Check sheet for the modelled part. Datum: model origin and axes. Units: mm. Coordinates: 2 decimals unless noted, no trailing zeros. Order: outer loops, then holes, each group sorted by start corner. A loop starts at its lowest first (then second) coordinate and runs counter-clockwise, first axis right, second up.
1. Cross-section at C-C (x = 0). Enter the section's corners in (y, z) (1 decimal).
2. Cross-section at D-D (y = 190.5). Enter the section's corners in (x, z) (1 decimal), then the cut area to 3 significant figures.
3. Cross-section at A-A (z = 0). Enter the section's corners in (x, y) (1 decimal).
4. Cross-section at B-B (y = 6.35). Enter the section's corners in (x, z) (1 decimal).
5. Gauge pin test, flat ends, axial feed: pin 1 Ø1 at (y, z) = (171, -1) entering from -X; pin 2 Ø1.5 at (y, z) = (73.5, 3.5) entering from -X; pin 3 Ø1 at (x, z) = (0.5, 0.5) entering from -Y. Record the tip position at first contact, or that the pin passes through.
6. Thickness scan on line 1 (Y direction, x = -2.85, z = 0) (3 decimals); line 2 (X direction, y = 111, z = 1.5); line 3 (X direction, y = 114.5, z = 0.25). Record the ranges inside material, lowest first.
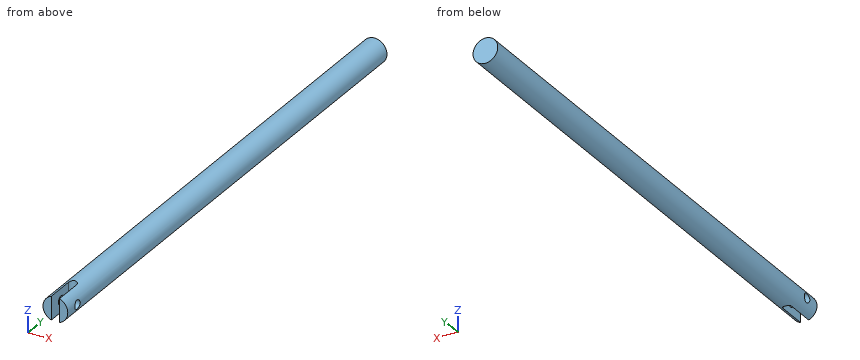
```python
from build123d import *

# Parameters (mm, degrees)
SKETCH1_R               = 4.7625
BOSS_EXTRUDE1_DEPTH     = 206.375
CUT_EXTRUDE1_DEPTH      = 5.7625
CUT_EXTRUDE1_DEPTH_BACK = 5.7625
F_8_32_TAPPED_HOLE1_D   = 3.4544


with BuildPart() as part:
    # Sketch1 → Boss-Extrude1 (new body)
    with BuildSketch(Plane(origin=(0, 0, 0), x_dir=(1, 0, 0), z_dir=(0, 1, 0))):
        Circle(SKETCH1_R)
    extrude(amount=BOSS_EXTRUDE1_DEPTH)

    # Sketch2 → Cut-Extrude1 (cut, two sides)
    with BuildSketch(Plane.XY) as cut_extrude1_sk:
        with BuildLine():
            Line((-1.5875, -11.1125), (-1.5875, 11.1125))
            ThreePointArc((-1.5875, 11.1125), (0, 12.7), (1.5875, 11.1125))
            Line((1.5875, 11.1125), (1.5875, -11.1125))
            ThreePointArc((1.5875, -11.1125), (0, -12.7), (-1.5875, -11.1125))
        make_face()
    extrude(amount=CUT_EXTRUDE1_DEPTH, mode=Mode.SUBTRACT)
    extrude(cut_extrude1_sk.sketch, amount=-CUT_EXTRUDE1_DEPTH_BACK, mode=Mode.SUBTRACT)

    # #8-32 Tapped Hole1 (through all)
    with Locations(Plane(origin=(4.7625, 0, 0), x_dir=(0, 0, -1), z_dir=(1, 0, 0))):
        with Locations((0, 6.35)):
            Hole(F_8_32_TAPPED_HOLE1_D / 2)


solid = part.part
```
Data:
1. outline: (12.7, -4.8) - (206.4, -4.8) - (206.4, 4.8) - (12.7, 4.8) - close
2. outline: circle Ø9.5 at (0, 0)
2. area: 71.3 mm2
3. outline: (-4.8, 0) - (-1.6, 0) - (-1.6, 4.6) - (-4.8, 4.6) - close; (-4.8, 8.1) - (-1.6, 8.1) - (-1.6, 11.1) arc R1.6 cw to (1.6, 11.1) - (1.6, 8.1) - (4.8, 8.1) - (4.8, 206.4) - (-4.8, 206.4) - close; (1.6, 0) - (4.8, 0) - (4.8, 4.6) - (1.6, 4.6) - close
4. outline: (-4.4, -1.7) arc R4.8 ccw to (-1.6, -4.5) - (-1.6, -1.7) - close; (-4.4, 1.7) - (-1.6, 1.7) - (-1.6, 4.5) arc R4.8 ccw to start; (1.6, -4.5) arc R4.8 ccw to (4.4, -1.7) - (1.6, -1.7) - close; (1.6, 1.7) - (4.4, 1.7) arc R4.8 ccw to (1.6, 4.5) - close
5. pin 1: stops at x = -4.74
5. pin 2: stops at x = -3.89
5. pin 3: stops at y = 12.35
6. line 1: y = 0 to 4.623, 8.077 to 206.375
6. line 2: x = -4.52 to 4.52
6. line 3: x = -4.76 to 4.76
